```python
from build123d import *

# Parameters (mm, degrees)
F1_DEPTH    = 19.05
F2_T1_DEPTH = 171.45
F3_W        = 12.7
F3_H        = 38.1
F8_DEPTH    = 19.05
F9_R        = 5.08
F10_R       = 5.08
F11_R       = 5.08


# Not quite as in the source:
# - a fillet or chamfer that OpenCascade refuses, or shapes differently, is made with other operations: its cross-section is extruded or revolved along the edge and cut away or added


with BuildPart() as f1:
    # F0 (on Front) → F1 (new body, symmetric)
    with BuildSketch(Plane.XZ):
        Polygon((-38.1, 57.15), (-22.225, 0), (22.225, 0), (38.1, 57.15), (38.1, 101.6), (-38.1, 101.6), align=None)
    extrude(amount=F1_DEPTH, both=True)

    # F2: fillet of radius 19.05 on 2 edges, made by hand

    # F2_s2 → F2_t1 (cut)
    with BuildSketch(Plane.YZ.offset(-85.725)):
        with BuildLine():
            ThreePointArc((0, 101.6), (-13.4703841816, 96.0203841816), (-19.05, 82.55))
            Line((-19.05, 82.55), (-19.05, 101.6))
            Line((-19.05, 101.6), (0, 101.6))
        make_face()
        with BuildLine():
            ThreePointArc((0, 101.6), (13.4703841816, 96.0203841816), (19.05, 82.55))
            Line((19.05, 82.55), (19.05, 101.6))
            Line((19.05, 101.6), (0, 101.6))
        make_face()
    extrude(amount=F2_T1_DEPTH, mode=Mode.SUBTRACT)

    # F3 (on Front) → F4 (revolve)
    with BuildSketch(Plane.XZ):
        with Locations((6.35, 101.6)):
            Rectangle(F3_W, F3_H)
    revolve(axis=Axis((0, 0, 41.275), (0, 0, -1)))

    # F5 (on Right) → F6 (revolve)
    with BuildSketch(Plane.YZ):
        with BuildLine():
            Line((-5.08, 158.115), (-5.08, 102.235))
            add(Edge.make_bspline(
                [(-5.08, 102.235), (17.145, 102.235), (17.145, 130.175), (17.145, 158.115), (-5.08, 158.115)],
                knots=[3.1415926536, 3.1415926536, 3.1415926536, 4.7123889804, 4.7123889804, 6.2831853072, 6.2831853072, 6.2831853072], degree=2, weights=[1, 0.7071067812, 1, 0.7071067812, 1]))
        make_face()
    revolve(axis=Axis((0, -5.08, 55.275326029), (0, 0, -1)))

    # F7 (on face) → F8 (join)
    with BuildSketch(Plane.YZ.offset(38.1)):
        with BuildLine():
            Line((-23.622, 24.761857734), (14.5931466414, 70.3048960355))
            ThreePointArc((14.5931466414, 70.3048960355), (9.3486979196, 99.1483236264), (-18.0359002739, 88.6826015123))
            Line((-18.0359002739, 88.6826015123), (-30.8627206832, 50.9590916336))
            Line((-30.8627206832, 50.9590916336), (-74.213960244, 59.0636453196))
            Line((-74.213960244, 59.0636453196), (-79.2495722325, 45.6589880743))
            Line((-79.2495722325, 45.6589880743), (-23.622, 24.761857734))
        make_face()
    extrude(amount=F8_DEPTH)

    # F9
    f9_edges = [f1.edges().sort_by_distance(p)[0] for p in [
        (47.625, -30.862721, 50.959092),
    ]]
    fillet(f9_edges, radius=F9_R)

    # F10
    f10_edges = [f1.edges().sort_by_distance(p)[0] for p in [
        (47.625, -23.622, 24.761858),
    ]]
    fillet(f10_edges, radius=F10_R)

    # F11
    f11_edges = [f1.edges().sort_by_distance(p)[0] for p in [
        (57.15, -3.358654, 48.910773),
        (57.15, -53.118999, 35.842741),
        (57.15, -23.91241, 25.868412),
        (57.15, -54.701473, 55.415768),
        (57.15, -31.691239, 52.376034),
        (57.15, -23.740888, 71.904309),
        (57.15, 9.348698, 99.148324),
    ]]
    fillet(f11_edges, radius=F11_R)


solid = f1.part
```
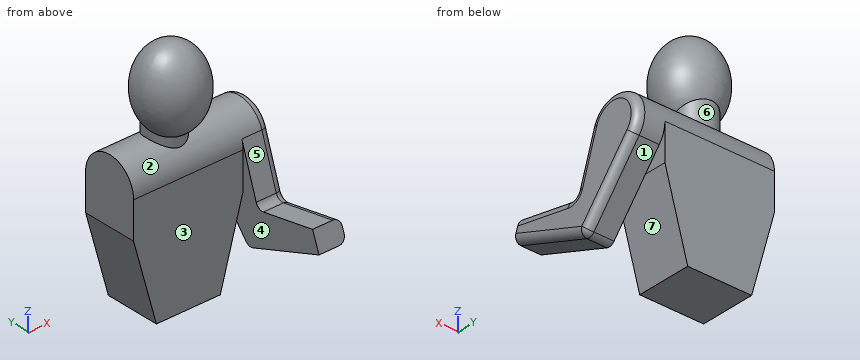
Part model, mm, in its own coordinate system. Face numbers are marked on the shaded views. A direction names the side the tool comes from. Round coordinates to 2 decimals unless told otherwise and drop trailing zeros. Use one line per item in the form item = value. Start each with the question number.
Item 1: Drop flat-ended pins along their axis: pin 1 Ø1.5 at (y, z) = (-3, 128.5) entering from -X; pin 2 Ø12 at (y, z) = (-34.5, 142) entering from -X. Give the stop position or say it passes through.
Item 2: Tool access for the marked faces 1, 2 and 3: list every direction of +Z, -Z, +X, -X, +Y, -Y with a clear straight run to the whole face (end or side of a thin tool).
Item 3: Two-plate mould, pull along X, no slides. Class the marked faces 4, 5, 6 and 7: released by +X, released by -X, zero draft, split by the parting line, or undercut.
Item 4: Drill centre lines: line 1 along Y through (x, z) = (5, 45); line 2 along X through (y, z) = (10, 62.5); line 3 along X through (y, z) = (-46, 43.5). Where is each one in solid material? Low to high.
Data:
q1.pin_1 = -22.15
q1.pin_2 = through
q2.face_1 = -Z, +X, +Y
q2.face_2 = none
q2.face_3 = -Z, -X, -Y
q3.face_4 = undercut
q3.face_5 = zero draft
q3.face_6 = split by the parting line
q3.face_7 = undercut
q4.line_1 = -19.05 to 19.05
q4.line_2 = -38.1 to 38.1
q4.line_3 = 38.1 to 57.15
